Job drawing, mm, ordinate dimensions from the low corner. One solid piece. Coordinates: 2 decimals unless noted, no trailing zeros. Write each loop counter-clockwise with the first axis right and the second up, starting at its lowest first coordinate (ties: lowest second). Pieces come first, ordered by that corner, then holes. Notation, with made-up numbers: (44.25, 11) - (86.25, 11) arc R7 ccw to (86.25, 16) - close; hole circle Ø3 at (37, -29). An arc over 180 degrees is marked (long way). Use one line per item in the form item = value. Start each with the question number.
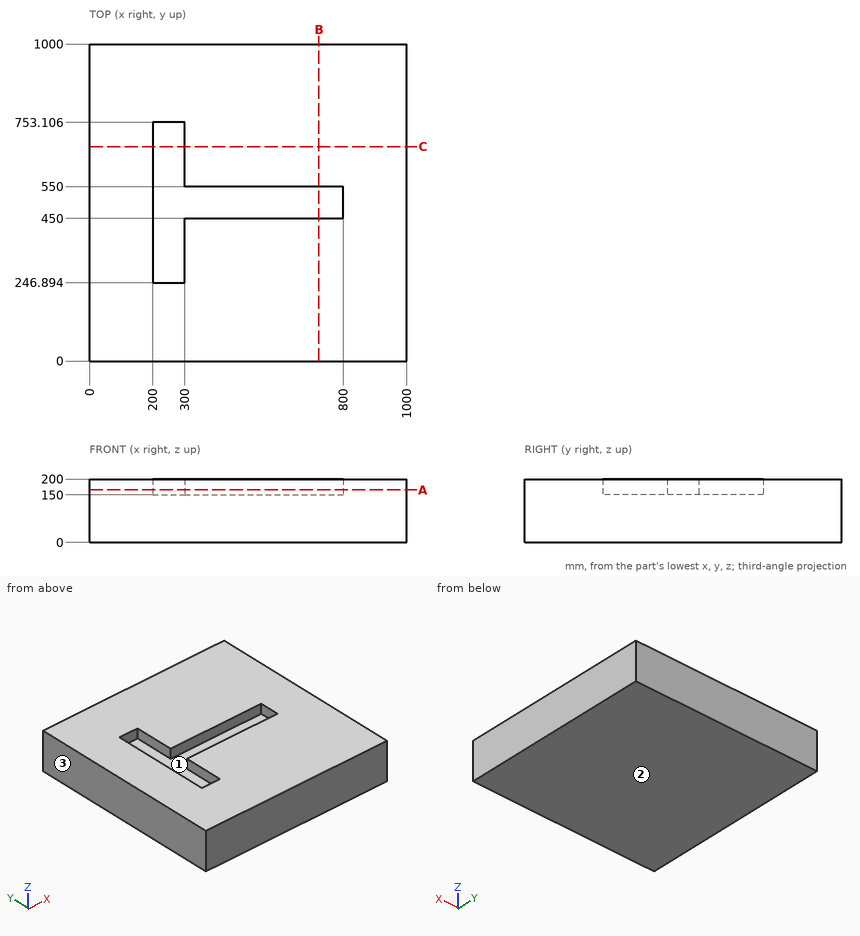
Q1. Slice it at B-B (x = 723.5). List the corners of the cut face in (y, z).
Q2. Drill centre lines: probe 1 along Y at (x, z) = (507.5, 177); probe 2 along X at (y, z) = (523, 178); probe 3 along Y at (x, z) = (205, 164). Where is each one in solid material? Low to high.
Q3. Slice it at A-A (z = 165.5). List the corners of the cut face in (x, y), plus the area to 3 significant figures.
Q4. Slice it at C-C (y = 676.5). List the corners of the cut face in (x, z).
Q5. Pin check, flat tip, straight feed: P1, Ø12, axis at x = 600, y = 364, coming from the -Z side. Stop position of the tip, or through.
Q6. Mould opens along X. For the marked faces 1, 2 and 3 say: released by +X, released by -X, zero draft, split by the parting line, or undercut.
Solution:
q1.outline = (0, 0) - (1000, 0) - (1000, 200) - (550, 200) - (550, 150) - (450, 150) - (450, 200) - (0, 200) - close
q2.probe_1 = 0 to 450, 550 to 1000
q2.probe_2 = 0 to 200, 800 to 1000
q2.probe_3 = 0 to 246.89, 753.11 to 1000
q3.outline = (0, 0) - (1000, 0) - (1000, 1000) - (0, 1000) - close; hole (200, 246.89) - (300, 246.89) - (300, 450) - (800, 450) - (800, 550) - (300, 550) - (300, 753.11) - (200, 753.11) - close
q3.area = 899,000 mm2
q4.outline = (0, 0) - (1000, 0) - (1000, 200) - (300, 200) - (300, 150) - (200, 150) - (200, 200) - (0, 200) - close
q5.P1 = 0
q6.face_1 = undercut
q6.face_2 = zero draft
q6.face_3 = released by -X
